from build123d import *

# Parameters (mm, degrees)
SKETCH1_R           = 2.4892
BOSS_EXTRUDE1_DEPTH = 3.175


with BuildPart() as part:
    # Sketch1 → Boss-Extrude1 (new body)
    with BuildSketch(Plane(origin=(0, 0, 0), x_dir=(-1, 0, 0), z_dir=(0, 0, -1))):
        with BuildLine():
            Line((-2.414213562, 0.585786438), (-0.585786438, 2.414213562))
            ThreePointArc((-0.585786438, 2.414213562), (-0.152240935, 3.06306026), (0, 3.828427125))
            Line((0, 3.828427125), (0, 72.371572875))
            ThreePointArc((0, 72.371572875), (-0.152240935, 73.13693974), (-0.585786438, 73.785786438))
            Line((-0.585786438, 73.785786438), (-2.414213562, 75.614213562))
            ThreePointArc((-2.414213562, 75.614213562), (-3.06306026, 76.047759065), (-3.828427125, 76.2))
            Line((-3.828427125, 76.2), (-21.571572875, 76.2))
            ThreePointArc((-21.571572875, 76.2), (-22.33693974, 76.047759065), (-22.985786438, 75.614213562))
            Line((-22.985786438, 75.614213562), (-24.814213562, 73.785786438))
            ThreePointArc((-24.814213562, 73.785786438), (-25.247759065, 73.13693974), (-25.4, 72.371572875))
            Line((-25.4, 72.371572875), (-25.4, 60.289301259))
            ThreePointArc((-25.4, 60.289301259), (-25.665349353, 58.682103933), (-26.433233299, 57.245494114))
            Line((-26.433233299, 57.245494114), (-30.162321659, 52.385651545))
            ThreePointArc((-30.162321659, 52.385651545), (-31.351237196, 51.272110628), (-32.834993135, 50.599829559))
            Line((-32.834993135, 50.599829559), (-56.961021847, 44.135279649))
            ThreePointArc((-56.961021847, 44.135279649), (-58.582132719, 43.975614164), (-60.168534235, 44.345511117))
            Line((-60.168534235, 44.345511117), (-65.827940772, 46.68971406))
            ThreePointArc((-65.827940772, 46.68971406), (-67.211252686, 47.549912686), (-68.24465063, 48.809111723))
            Line((-68.24465063, 48.809111723), (-74.285786438, 59.272665878))
            ThreePointArc((-74.285786438, 59.272665878), (-74.800314387, 59.859372559), (-75.500199155, 60.204517531))
            Line((-75.500199155, 60.204517531), (-77.997877056, 60.873768307))
            ThreePointArc((-77.997877056, 60.873768307), (-78.776567531, 60.924806377), (-79.515515147, 60.673967462))
            Line((-79.515515147, 60.673967462), (-94.88153011, 51.802394587))
            ThreePointArc((-94.88153011, 51.802394587), (-95.46823679, 51.287866637), (-95.813381762, 50.58798187))
            Line((-95.813381762, 50.58798187), (-96.482632539, 48.090303968))
            ThreePointArc((-96.482632539, 48.090303968), (-96.533670609, 47.311613493), (-96.282831694, 46.572665878))
            Line((-96.282831694, 46.572665878), (-62.011258818, -12.787439597))
            ThreePointArc((-62.011258818, -12.787439597), (-61.496730869, -13.374146278), (-60.796846101, -13.71929125))
            Line((-60.796846101, -13.71929125), (-58.2991682, -14.388542027))
            ThreePointArc((-58.2991682, -14.388542027), (-57.520477725, -14.439580097), (-56.78153011, -14.188741182))
            Line((-56.78153011, -14.188741182), (-38.670072037, -3.732085988))
            ThreePointArc((-38.670072037, -3.732085988), (-38.083489199, -3.442815344), (-37.464167262, -3.232583875))
            Line((-37.464167262, -3.232583875), (-26.035832738, -0.170370869))
            ThreePointArc((-26.035832738, -0.170370869), (-25.394368473, -0.042775693), (-24.741737512, 0))
            Line((-24.741737512, 0), (-3.828427125, 0))
            ThreePointArc((-3.828427125, 0), (-3.06306026, 0.152240935), (-2.414213562, 0.585786438))
        make_face()
        with Locations((-12.7, 12.7)):
            Circle(SKETCH1_R, mode=Mode.SUBTRACT)
        with Locations((-61.798522628, 12.244090512)):
            Circle(SKETCH1_R, mode=Mode.SUBTRACT)
        with Locations((-74.498522628, 34.241135768)):
            Circle(SKETCH1_R, mode=Mode.SUBTRACT)
        with Locations((-12.7, 25.4)):
            Circle(SKETCH1_R, mode=Mode.SUBTRACT)
        with Locations((-80.848522628, 45.239658396)):
            Circle(SKETCH1_R, mode=Mode.SUBTRACT)
        with Locations((-68.148522628, 23.24261314)):
            Circle(SKETCH1_R, mode=Mode.SUBTRACT)
        with Locations((-55.448522628, 1.245567884)):
            Circle(SKETCH1_R, mode=Mode.SUBTRACT)
        with Locations((-12.7, 38.1)):
            Circle(SKETCH1_R, mode=Mode.SUBTRACT)
        with Locations((-30.825461194, 31.649870813)):
            Circle(SKETCH1_R, mode=Mode.SUBTRACT)
        with Locations((-12.7, 50.8)):
            Circle(SKETCH1_R, mode=Mode.SUBTRACT)
        with Locations((-12.7, 63.5)):
            Circle(SKETCH1_R, mode=Mode.SUBTRACT)
        with Locations((-49.226348185, 26.719368004)):
            Circle(SKETCH1_R, mode=Mode.SUBTRACT)
        with Locations((-37.560653285, 19.984175913)):
            Circle(SKETCH1_R, mode=Mode.SUBTRACT)
        with Locations((-34.074261314, 6.972783942)):
            Circle(SKETCH1_R, mode=Mode.SUBTRACT)
        with BuildLine():
            Line((-43.451427823, 32.351315517), (-44.895538661, 37.740810537))
            ThreePointArc((-44.895538661, 37.740810537), (-43.135408461, 40.789445471), (-40.086773527, 39.029315271))
            Line((-40.086773527, 39.029315271), (-38.642662689, 33.639820251))
            ThreePointArc((-38.642662689, 33.639820251), (-40.402792889, 30.591185317), (-43.451427823, 32.351315517))
        make_face(mode=Mode.SUBTRACT)
    extrude(amount=-BOSS_EXTRUDE1_DEPTH)


solid = part.part
The model under review builds one solid part; all positions refer to its coordinate system, in mm. A direction names the side the tool comes from. Round coordinates to 2 decimals unless told otherwise and drop trailing zeros. Order: outer loops, then holes, each group sorted by start corner. A loop starts at its lowest first (then second) coordinate and runs counter-clockwise, first axis right, second up. Notation, with made-up numbers: (1, -4) -> (32, -4) arc R22 ccw to (32, 11) -> close; hole circle Ø8 at (-5, 37.25). An arc over 180 degrees is marked (long way). Use CSV: the item, a comma, the result in double quotes. Start each with the question number.
(1) Consider section C-C on x = 49. Write out the cut boundary in (y, z) (3 decimals).
(2) Wall thickness on probe 1 along Y at (x, z) = (13.5, 1.7); probe 2 along X at (y, z) = (36, 0.8); probe 3 along Y at (x, z) = (9.5, 0.25): over which ranges is each line inside the solid? List them lowest first. Write a range as from..to.
(3) Tool access review of faces 4 (the face through (44.163, 35.008, 1.565)), 5 (the face through (76.732, 60.534, 1.565)), 6 (the face through (87.09, 56.3, 1.57)): name each direction out of +Z, -Z, +X, -X, +Y, -Y from which nothing blocks a thin tool from reaching the whole face with its end or side.
(4) Mouldability with a two-part tool opening along X and no side actions: class faces 1 (the face through (0, 38, 2)), 2 (the face through (83.335, 45.349, 1.565)), 3 (the face through (59.57, -14.05, 1.57)) as pulls with the +X half, pulls with the -X half, needs draft (parallel to the pull), parting line crosses it, or undercut.
(5) Consider section D-D on z = 1.15. State how many separate pieces and enclosed holes the cut face has, and give its area (3 significant figures).
(6) Consider section A-A on x = 12.7. Write out the cut boundary in (y, z) (3 decimals).
(7) Consider section B-B on y = 63.5. Write out the cut boundary in (x, z) (3 decimals).
Responses:
1,outline,"(-9.696, 0) -> (24.24, 0) -> (24.24, 3.175) -> (-9.696, 3.175) -> close; (29.198, 0) -> (46.268, 0) -> (46.268, 3.175) -> (29.198, 3.175) -> close"
2,probe 1,"0..10.34, 15.06..23.04, 27.76..35.74, 40.46..48.44, 53.16..61.14, 65.86..76.2"
2,probe 2,"0..11.36, 14.04..39.28, 44.43..72.74, 76.26..90.18"
2,probe 3,"0..76.2"
3,face 4,"+Z, -Z"
3,face 5,"+Z, -Z, +Y"
3,face 6,"+Z, -Z, +X, +Y"
4,face 1,"pulls with the -X half"
4,face 2,"undercut"
4,face 3,"pulls with the +X half"
5,separate pieces,"1"
5,enclosed holes,"15"
5,area,"4,920 mm²"
6,outline,"(0, 0) -> (10.211, 0) -> (10.211, 3.175) -> (0, 3.175) -> close; (15.189, 0) -> (22.911, 0) -> (22.911, 3.175) -> (15.189, 3.175) -> close; (27.889, 0) -> (35.611, 0) -> (35.611, 3.175) -> (27.889, 3.175) -> close; (40.589, 0) -> (48.311, 0) -> (48.311, 3.175) -> (40.589, 3.175) -> close; (53.289, 0) -> (61.011, 0) -> (61.011, 3.175) -> (53.289, 3.175) -> close; (65.989, 0) -> (76.2, 0) -> (76.2, 3.175) -> (65.989, 3.175) -> close"
7,outline,"(0, 0) -> (10.211, 0) -> (10.211, 3.175) -> (0, 3.175) -> close; (15.189, 0) -> (25.4, 0) -> (25.4, 3.175) -> (15.189, 3.175) -> close"
